Here's how the part is built. I have some questions about the finished solid (model axes, mm). Round coordinates to 2 decimals unless told otherwise and drop trailing zeros. Write each loop counter-clockwise with the first axis right and the second up, starting at its lowest first coordinate (ties: lowest second). Pieces come first, ordered by that corner, then holes. Notation, with made-up numbers: M -20,57.25 L 17,57.25 A14 ccw 17,82.25 Z; hole C 74.5,-15 d3. An arc over 180 degrees is marked long. Write item = value, one per line. Start each with the question number.
(1) I need wall thicknesses on line 1 along Y through (x, z) = (-25, 1.8); line 2 along Y through (x, z) = (6, 1.3); line 3 along X through (y, z) = (29.5, 0.2). Which ranges of each line are inside material? Lowest first, please.
(2) Will these pins go through, and if not, where does the flat tip stop? pin 1 Ø3 at (x, y) = (-22, 10) entering from -Z; pin 2 Ø1 at (y, z) = (-27, 1.5) entering from +X.
(3) I want a section at B-B (z = 1.9). List the corners of the cut face in (x, y) for me, and give its area (3 significant figures).
(4) I want a section at A-A (y = 0). List the corners of the cut face in (x, z) for me.
(5) I want a section at C-C (x = 0). List the corners of the cut face in (y, z) for me, and give its area (3 significant figures).
```python
from build123d import *

# Parameters (mm, degrees)
F0_R         = 27.1053686487
F1_DEPTH     = 2.794
F2_T2_ANGLE  = 130.513894387
F2_T4_ANGLE  = 343.3509048615
F2_T6_ANGLE  = 130.513894387
F2_T8_ANGLE  = 343.3509048615
F2_T10_ANGLE = 130.513894387
F2_T12_ANGLE = 343.3509048615


# Not quite as in the source:
# - a fillet or chamfer that OpenCascade refuses, or shapes differently, is made with other operations: its cross-section is extruded or revolved along the edge and cut away or added


with BuildPart() as f1:
    # F0 (on Top) → F1 (new body)
    with BuildSketch(Plane.XY):
        with BuildLine():
            ThreePointArc((39.4058168676, -14.1300394968), (41.2438235607, -7.1710136852), (41.8625897333, 0))
            ThreePointArc((41.8625897333, 0), (32.1326921102, 26.8321918026), (7.4659352731, 41.1914582126))
            ThreePointArc((7.4659352731, 41.1914582126), (0, 34.366550311), (-7.4659352731, 41.1914582126))
            ThreePointArc((-7.4659352731, 41.1914582126), (-36.2540661773, 20.9312948667), (-39.4058168676, -14.1300394968))
            ThreePointArc((-39.4058168676, -14.1300394968), (-32.218910691, -14.6140069025), (-28.758026755, -20.9312948667))
            ThreePointArc((-28.758026755, -20.9312948667), (-29.6008750359, -24.3846489835), (-31.9398815945, -27.0614187158))
            ThreePointArc((-31.9398815945, -27.0614187158), (0, -41.8625897333), (31.9398815945, -27.0614187158))
            ThreePointArc((31.9398815945, -27.0614187158), (29.7623056098, -17.1832751555), (39.4058168676, -14.1300394968))
        make_face()
        Circle(F0_R, mode=Mode.SUBTRACT)
    extrude(amount=F1_DEPTH)

    # F2: fillet of radius 5.08 on 6 edges, made by hand

    # F2_s1 → F2_t2 (revolve, cut)
    with BuildSketch(Plane(origin=(0, 0, 0), x_dir=(0, 0, 1), z_dir=(0.9957938256, -0.0916223607, 0))):
        with BuildLine():
            ThreePointArc((2.794, -37.3260046741), (2.0394641369, -39.9899791484), (0, -41.8625897333))
            Line((0, -41.8625897333), (2.794, -41.8625897333))
            Line((2.794, -41.8625897333), (2.794, -37.3260046741))
        make_face()
    revolve(axis=Axis((0, 0, 2.794), (0, 0, 1)), revolution_arc=F2_T2_ANGLE, mode=Mode.SUBTRACT)

    # F2_s3 → F2_t4 (revolve, cut)
    with BuildSketch(Plane(origin=(3.7584385128, 4.7548188772, 0), x_dir=(0, 0, 1), z_dir=(0.6201152013, 0.7845107629, 0))):
        with BuildLine():
            ThreePointArc((0, 48.9175586674), (2.0394641369, 50.7901692523), (2.794, 53.4541437266))
            Line((2.794, 53.4541437266), (2.794, 48.9175586674))
            Line((2.794, 48.9175586674), (0, 48.9175586674))
        make_face()
    revolve(axis=Axis((36.2540661773, -20.9312948667, 2.794), (0, 0, -1)), revolution_arc=F2_T4_ANGLE, mode=Mode.SUBTRACT)

    # F2_s5 → F2_t6 (revolve, cut)
    with BuildSketch(Plane(origin=(0, 0, 0), x_dir=(0, 0, 1), z_dir=(-0.4185496208, 0.9081939302, 0))):
        with BuildLine():
            ThreePointArc((2.794, -37.3260046741), (2.0394641369, -39.9899791484), (0, -41.8625897333))
            Line((0, -41.8625897333), (2.794, -41.8625897333))
            Line((2.794, -41.8625897333), (2.794, -37.3260046741))
        make_face()
    revolve(axis=Axis((0, 0, 2.794), (0, 0, 1)), revolution_arc=F2_T6_ANGLE, mode=Mode.SUBTRACT)

    # F2_s7 → F2_t8 (revolve, cut)
    with BuildSketch(Plane(origin=(-3.7584385128, 4.7548188772, 0), x_dir=(0, 0, 1), z_dir=(-0.6201152013, 0.7845107629, 0))):
        with BuildLine():
            ThreePointArc((2.794, -53.4541437266), (2.0394641369, -50.7901692523), (0, -48.9175586674))
            Line((0, -48.9175586674), (2.794, -48.9175586674))
            Line((2.794, -48.9175586674), (2.794, -53.4541437266))
        make_face()
    revolve(axis=Axis((-36.2540661773, -20.9312948667, 2.794), (0, 0, 1)), revolution_arc=F2_T8_ANGLE, mode=Mode.SUBTRACT)

    # F2_s9 → F2_t10 (revolve, cut)
    with BuildSketch(Plane(origin=(0, 0, 0), x_dir=(0, 0, 1), z_dir=(-0.9957938256, -0.0916223607, 0))):
        with BuildLine():
            ThreePointArc((2.794, 37.3260046741), (2.0394641369, 39.9899791484), (0, 41.8625897333))
            Line((0, 41.8625897333), (2.794, 41.8625897333))
            Line((2.794, 41.8625897333), (2.794, 37.3260046741))
        make_face()
    revolve(axis=Axis((0, 0, 2.794), (0, 0, -1)), revolution_arc=F2_T10_ANGLE, mode=Mode.SUBTRACT)

    # F2_s11 → F2_t12 (revolve, cut)
    with BuildSketch(Plane(origin=(-5.9970131945, 0.877493792, 0), x_dir=(0, 0, 1), z_dir=(-0.9894638509, 0.1447801361, 0))):
        with BuildLine():
            ThreePointArc((2.794, 53.4541437266), (2.0394641369, 50.7901692523), (0, 48.9175586674))
            Line((0, 48.9175586674), (2.794, 48.9175586674))
            Line((2.794, 48.9175586674), (2.794, 53.4541437266))
        make_face()
    revolve(axis=Axis((0, 41.8625897333, 2.794), (0, 0, -1)), revolution_arc=F2_T12_ANGLE, mode=Mode.SUBTRACT)


solid = f1.part
```
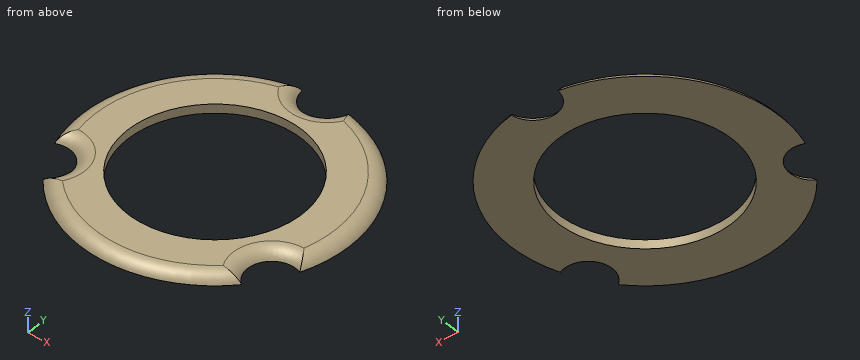
Returned:
q1.line_1 = -31.67 to -10.47, 10.47 to 31.67
q1.line_2 = -40.48 to -26.43, 26.43 to 35.93
q1.line_3 = -29.55 to 29.55
q2.pin_1 = through
q2.pin_2 = 30.95
q3.outline = M -38.36,-12.02 A9.15 cw -29.59,-27.21 A40.2 ccw 29.59,-27.21 A9.15 cw 38.36,-12.02 A40.2 ccw 8.77,39.24 A9.15 cw -8.77,39.24 A40.2 ccw Z; hole C 0,0 d54.21
q3.area = 2,480 mm²
q4.outline = M -41.86,0 L -27.11,0 L -27.11,2.79 L -37.33,2.79 A5.08 ccw Z; M 27.11,0 L 41.86,0 A5.08 ccw 37.33,2.79 L 27.11,2.79 Z
q5.outline = M -41.86,0 L -27.11,0 L -27.11,2.79 L -37.33,2.79 A5.08 ccw Z; M 27.11,0 L 34.37,0 A5.08 ccw 29.83,2.79 L 27.11,2.79 Z
q5.area = 54.3 mm²
